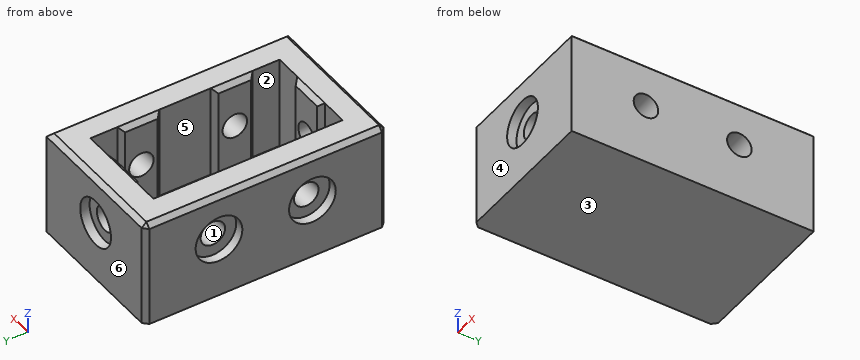
Autodesk Fusion 360 part; units mm, degrees
sketch "Main Profile" plane through (0, 0, 0) normal (0, 0, 1) x (1, 0, 0)
  line L0 (10.25, -20.25) -> (-10.25, -20.25)
  line L1 (-10.25, -20.25) -> (-10.25, 20.25)
  line L2 (-10.25, 20.25) -> (10.25, 20.25)
  line L3 (10.25, 20.25) -> (10.25, -20.25)
  line L4 (10.25, -20.25) -> (-10.25, 20.25) construction
  line L5 (-10.25, -20.25) -> (10.25, 20.25) construction
  line L6 (-16, -25.9) -> (16, -25.9)
  line L7 (16, -25.9) -> (16, 25.9)
  line L8 (16, 25.9) -> (-16, 25.9)
  line L9 (-16, 25.9) -> (-16, -25.9)
  line L10 (-16, -25.9) -> (16, 25.9) construction
  line L11 (16, -25.9) -> (-16, 25.9) construction
  line L12 (-3.5, 19.25) -> (3.5, 19.25)
  line L13 (3.5, 19.25) -> (4.5, 20.25)
  line L14 (-3.5, 19.25) -> (-4.5, 20.25)
  line L15 (0, 20.25) -> (0, 19.25) construction
  line L16 (-9.25, 6.5) -> (-9.25, 13.5)
  line L17 (-9.25, 13.5) -> (-10.25, 14.5)
  line L18 (-9.25, 6.5) -> (-10.25, 5.5)
  line L19 (9.25, 13.5) -> (9.25, 6.5)
  line L20 (9.25, 6.5) -> (10.25, 5.5)
  line L21 (9.25, 13.5) -> (10.25, 14.5)
  line L22 (9.25, -13.5) -> (10.25, -14.5)
  line L23 (9.25, -6.5) -> (9.25, -13.5)
  line L24 (9.25, -6.5) -> (10.25, -5.5)
  line L25 (3.5, -19.25) -> (4.5, -20.25)
  line L26 (3.5, -19.25) -> (-3.5, -19.25)
  line L27 (-3.5, -19.25) -> (-4.5, -20.25)
  line L28 (-9.25, -13.5) -> (-10.25, -14.5)
  line L29 (-9.25, -13.5) -> (-9.25, -6.5)
  line L30 (-9.25, -6.5) -> (-10.25, -5.5)
  point P0 (0, 10)
  dimension "d1" = 40.5
  dimension "d2" = 20.5
  dimension "d3" = 32
  dimension "d4" = 51.8
  dimension "d5" = 1
  dimension "d6" = 135
  dimension "d7" = 7
  dimension "d8" = 135
  dimension "d9" = 10.25
  dimension "d11" = 360
  dimension "d13" = 360
extrude "Extrude1" add sketch "Main Profile" along normal blind 3 contours L0 L1 L2 L3 L12 L13 L14 L16 L17 L18 L19 L20 L21 L22 L23 L24 L25 L26 L27 L28 L29 L30 | L0 L25 L26 L27 | L3 L22 L23 L24 | L3 L19 L20 L21 | L1 L28 L29 L30 | L1 L16 L17 L18 | L2 L12 L13 L14 | L6 L7 L8 L9
extrude "Extrude2" add sketch "Main Profile" along normal blind 22.9 contours L0 L25 L26 L27 | L3 L22 L23 L24 | L3 L19 L20 L21 | L1 L28 L29 L30 | L1 L16 L17 L18 | L2 L12 L13 L14 | L6 L7 L8 L9
sketch "Short Side" plane through (0, 25.9, 0) normal (0, 1, 0) x (-1, 0, 0)
  line L0 (-16, 0) -> (16, 0)
  line L1 (16, 0) -> (16, 22.9)
  line L2 (16, 22.9) -> (-16, 22.9)
  line L3 (-16, 22.9) -> (-16, 0)
  circle A0 centre (0, 12.9) radius 5
  circle A1 centre (0, 12.9) radius 2.625
  dimension "d18" = 10
  dimension "d19" = 5.25
  dimension "d20" = 12.9
extrude "Extrude3" cut sketch "Short Side" against normal blind 63.819 contours A1
extrude "Extrude4" cut sketch "Short Side" against normal blind 2 contours A0
extrude "Extrude5" cut sketch "Short Side" along normal blind 2 from surface at -51.8 contours A0
sketch "Long Side" plane through (-16, 0, 0) normal (-1, 0, 0) x (0, -1, 0)
  line L0 (-25.9, 0) -> (25.9, 0)
  line L1 (25.9, 0) -> (25.9, 22.9)
  line L2 (25.9, 22.9) -> (-25.9, 22.9)
  line L3 (-25.9, 22.9) -> (-25.9, 0)
  circle A0 centre (-10, 12.9) radius 5
  circle A1 centre (-10, 12.9) radius 2.625
  circle A2 centre (10, 12.9) radius 5
  circle A3 centre (10, 12.9) radius 2.625
  dimension "d28" = 10
  dimension "d29" = 5.25
  dimension "d30" = 10
  dimension "d31" = 12.9
  dimension "d34" = 20
  dimension "d35" = 0
extrude "Extrude6" cut sketch "Long Side" against normal blind 62.946 contours A1 | A3
extrude "Extrude7" cut sketch "Long Side" against normal blind 2 contours A0 | A2
chamfer "Chamfer1" distance 1 angle 45 12 edges at (9.25, 10, 22.9) (9.25, -10, 22.9) (-9.25, -10, 22.9) (0, -19.25, 22.9) (-9.25, 10, 22.9) (0, 19.25, 22.9) (0, 25.9, 22.9) (16, 0, 22.9) (0, -25.9, 22.9) (-16, 0, 22.9) (-16, -25.9, 11.45) (-16, 25.9, 11.45)
CAD build for the part. Positions are in the model's coordinates, mm. Face numbers are marked on the shaded views. A direction names the side the tool comes from. Give positions to 0.01 mm unless a question says otherwise; leave off trailing zeros. Loops run counter-clockwise (first coordinate to the right, second up) from the corner with the lowest first, then second, coordinate; pieces in that order, holes last. Notation, with made-up numbers: M 14.25,5.25 L 46.25,5.25 A3 ccw 46.25,10.25 Z; hole C 27.5,44 d6. An arc over 180 degrees is marked long. Answer in a Markdown table with one row per item. Add a question column.
Item 1: Probe probe 1 along X at (y, z) = (2, 14); probe 2 along Z at (x, y) = (0, -24.35); probe 3 along Y at (x, z) = (7, 16.5). List the from-to ranges inside material, lowest first.
Item 2: Drop flat-ended pins along their axis: P1, Ø8, axis at y = -10, z = 12.9, coming from the -X side; P2, Ø12, axis at x = -1.5, y = 4.5, coming from the +Z side; P3, Ø2, axis at x = 1.5, z = 10.5, coming from the +Y side. Give the stop position or say it passes through.
Item 3: Mould opens along Y. For the marked faces 3, 4, 5 and 6 say: +Y half, -Y half, draft (parallel to the pull), parting line (faces both ways), or undercut.
Item 4: Band-saw the part on D-D on y = -16. Give the cut face in (x, z).
Item 5: Band-saw the part on A-A on x = 0. Give the cut face in (y, z) (3 decimals).
Item 6: Tool access for the marked faces 1 and 2: list every direction of +Z, -Z, +X, -X, +Y, -Y with a clear straight run to the whole face (end or side of a thin tool).
Item 7: Band-saw the part on C-C on y = -10. Give the cut face in (x, z) (3 decimals), then the cut area to 3 significant figures.
Reply:
| question | item | result |
|---|---|---|
| 1 | probe 1 | x = -16 to -10.25, 10.25 to 16 |
| 1 | probe 2 | z = 0 to 7.9, 17.9 to 22.9 |
| 1 | probe 3 | y = -25.9 to -20.25, 20.25 to 25.9 |
| 2 | P1 | stops at x = -14 |
| 2 | P2 | stops at z = 3 |
| 2 | P3 | stops at y = 23.9 |
| 3 | face 3 | draft |
| 3 | face 4 | -Y half |
| 3 | face 5 | undercut |
| 3 | face 6 | +Y half |
| 4 | outline | M -16,0 L 16,0 L 16,21.9 L 15,22.9 L 10.25,22.9 L 10.25,3 L -10.25,3 L -10.25,22.9 L -15,22.9 L -16,21.9 Z |
| 5 | outline | M -25.9,0 L 25.9,0 L 25.9,7.9 L 23.9,7.9 L 23.9,10.275 L 19.25,10.275 L 19.25,3 L -19.25,3 L -19.25,10.275 L -23.9,10.275 L -23.9,7.9 L -25.9,7.9 Z; M -25.9,17.9 L -23.9,17.9 L -23.9,15.525 L -19.25,15.525 L -19.25,21.9 L -20.25,22.9 L -24.9,22.9 L -25.9,21.9 Z; M 19.25,15.525 L 23.9,15.525 L 23.9,17.9 L 25.9,17.9 L 25.9,21.9 L 24.9,22.9 L 20.25,22.9 L 19.25,21.9 Z |
| 6 | face 1 | +X, -X |
| 6 | face 2 | +Z |
| 7 | outline | M -16,0 L 16,0 L 16,10.275 L 9.25,10.275 L 9.25,3 L -9.25,3 L -9.25,10.275 L -14,10.275 L -14,7.9 L -16,7.9 Z; M -16,17.9 L -14,17.9 L -14,15.525 L -9.25,15.525 L -9.25,21.9 L -10.25,22.9 L -15,22.9 L -16,21.9 Z; M 9.25,15.525 L 16,15.525 L 16,21.9 L 15,22.9 L 10.25,22.9 L 9.25,21.9 Z |
| 7 | area | 282 mm^2 |
